Here's how the part is built. I have some questions about the finished solid (model axes, mm). Round coordinates to 2 decimals unless told otherwise and drop trailing zeros. Use one line per item in the form item = value. Start each with the question number.
1. Will these pins go through, and if not, where does the flat tip stop? pin 1 (4 mm diameter, centred on y = 1.5, z = 383, fed in from -X); pin 2 (1.8 mm diameter, centred on x = 2.5, z = 310.5, fed in from +Y); pin 3 (2 mm diameter, centred on x = 4.5, z = 294.5, fed in from -Y).
2. I want a section at A-A, the plane z = 497. State how many separate pieces and enclosed holes the cut face has, plus the area to 3 significant figures.
3. If I drill on line 1 along X through (y, z) = (6.5, 167); line 2 along X through (y, z) = (-1.75, 24.5); line 3 along X through (y, z) = (7.5, 254.5), over which ranges is the centre line in solid material (lowest first)?
```python
from build123d import *

# Parameters (mm, degrees)
EXTRUDE1_DEPTH = 574


with BuildPart() as part:
    # Sketch1 → Extrude1 (new body)
    with BuildSketch(Plane.XY):
        with BuildLine():
            Line((3.232233116, 4.565447254), (0.953589838, 4.565447254))
            ThreePointArc((0.953589838, 4.565447254), (0.901826028, 4.558632419), (0.853589836, 4.538652333))
            Line((0.853589836, 4.538652333), (0.100000003, 4.103567024))
            ThreePointArc((0.100000003, 4.103567024), (0, 4.076772104), (-0.100000003, 4.103567024))
            Line((-0.100000003, 4.103567024), (-0.853589836, 4.538652333))
            ThreePointArc((-0.853589836, 4.538652333), (-0.901826028, 4.558632419), (-0.953589838, 4.565447254))
            Line((-0.953589838, 4.565447254), (-3.232233116, 4.565447254))
            ThreePointArc((-3.232233116, 4.565447254), (-3.417445277, 4.601015929), (-3.576306433, 4.702661433))
            Line((-3.576306433, 4.702661433), (-5.844073317, 6.853456827))
            ThreePointArc((-5.844073317, 6.853456827), (-5.959367314, 7.018804885), (-6, 7.216242649))
            Line((-6, 7.216242649), (-6, 7.948478858))
            ThreePointArc((-6, 7.948478858), (-5.855954134, 8.296236342), (-5.50819665, 8.440282208))
            Line((-5.50819665, 8.440282208), (-3.49180335, 8.440282208))
            ThreePointArc((-3.49180335, 8.440282208), (-3.144045866, 8.584328074), (-3, 8.932085558))
            Line((-3, 8.932085558), (-3, 9.249999634))
            ThreePointArc((-3, 9.249999634), (-3.058578644, 9.39142099), (-3.2, 9.449999634))
            Line((-3.2, 9.449999634), (-3.350000366, 9.449999634))
            ThreePointArc((-3.350000366, 9.449999634), (-3.491421722, 9.508578278), (-3.550000366, 9.649999634))
            Line((-3.550000366, 9.649999634), (-3.550000366, 9.8))
            ThreePointArc((-3.550000366, 9.8), (-3.60857901, 9.941421356), (-3.750000366, 10))
            Line((-3.750000366, 10), (-8.50000115, 10))
            ThreePointArc((-8.50000115, 10), (-9.560660508, 9.560660508), (-10, 8.50000115))
            Line((-10, 8.50000115), (-10, 7))
            ThreePointArc((-10, 7), (-5.02081528, -5.02081528), (7, -10))
            Line((7, -10), (8.50000115, -10))
            ThreePointArc((8.50000115, -10), (9.560660508, -9.560660508), (10, -8.50000115))
            Line((10, -8.50000115), (10, -3.750000366))
            ThreePointArc((10, -3.750000366), (9.941421356, -3.60857901), (9.8, -3.550000366))
            Line((9.8, -3.550000366), (9.649999634, -3.550000366))
            ThreePointArc((9.649999634, -3.550000366), (9.508578278, -3.491421722), (9.449999634, -3.350000366))
            Line((9.449999634, -3.350000366), (9.449999634, -3.2))
            ThreePointArc((9.449999634, -3.2), (9.39142099, -3.058578644), (9.249999634, -3))
            Line((9.249999634, -3), (8.866638303, -3))
            ThreePointArc((8.866638303, -3), (8.518880819, -3.144045866), (8.374834953, -3.49180335))
            Line((8.374834953, -3.49180335), (8.374834953, -5.50819665))
            ThreePointArc((8.374834953, -5.50819665), (8.230789087, -5.855954134), (7.883031603, -6))
            Line((7.883031603, -6), (7.150795394, -6))
            ThreePointArc((7.150795394, -6), (6.95335763, -5.959367314), (6.788009572, -5.844073317))
            Line((6.788009572, -5.844073317), (4.637214178, -3.576306432))
            ThreePointArc((4.637214178, -3.576306432), (4.535568675, -3.417445276), (4.5, -3.232233115))
            Line((4.5, -3.232233115), (4.5, -0.953589838))
            ThreePointArc((4.5, -0.953589838), (4.493185165, -0.901826026), (4.473205078, -0.853589834))
            Line((4.473205078, -0.853589834), (4.038119764, -0.100000004))
            ThreePointArc((4.038119764, -0.100000004), (4.011324842, 0), (4.038119764, 0.100000004))
            Line((4.038119764, 0.100000004), (4.473205078, 0.853589834))
            ThreePointArc((4.473205078, 0.853589834), (4.493185165, 0.901826026), (4.5, 0.953589838))
            Line((4.5, 0.953589838), (4.5, 3.232233115))
            ThreePointArc((4.5, 3.232233115), (4.535568675, 3.417445276), (4.637214178, 3.576306432))
            Line((4.637214178, 3.576306432), (6.788009572, 5.844073317))
            ThreePointArc((6.788009572, 5.844073317), (6.95335763, 5.959367314), (7.150795394, 6))
            Line((7.150795394, 6), (7.883031603, 6))
            ThreePointArc((7.883031603, 6), (8.230789087, 5.855954134), (8.374834953, 5.50819665))
            Line((8.374834953, 5.50819665), (8.374834953, 3.49180335))
            ThreePointArc((8.374834953, 3.49180335), (8.518880819, 3.144045866), (8.866638303, 3))
            Line((8.866638303, 3), (9.249999634, 3))
            ThreePointArc((9.249999634, 3), (9.39142099, 3.058578644), (9.449999634, 3.2))
            Line((9.449999634, 3.2), (9.449999634, 3.350000366))
            ThreePointArc((9.449999634, 3.350000366), (9.508578278, 3.491421722), (9.649999634, 3.550000366))
            Line((9.649999634, 3.550000366), (9.8, 3.550000366))
            ThreePointArc((9.8, 3.550000366), (9.941421356, 3.60857901), (10, 3.750000366))
            Line((10, 3.750000366), (10, 8.50000115))
            ThreePointArc((10, 8.50000115), (9.560660508, 9.560660508), (8.50000115, 10))
            Line((8.50000115, 10), (3.750000366, 10))
            ThreePointArc((3.750000366, 10), (3.60857901, 9.941421356), (3.550000366, 9.8))
            Line((3.550000366, 9.8), (3.550000366, 9.649999634))
            ThreePointArc((3.550000366, 9.649999634), (3.491421722, 9.508578278), (3.350000366, 9.449999634))
            Line((3.350000366, 9.449999634), (3.2, 9.449999634))
            ThreePointArc((3.2, 9.449999634), (3.058578644, 9.39142099), (3, 9.249999634))
            Line((3, 9.249999634), (3, 8.932085558))
            ThreePointArc((3, 8.932085558), (3.144045866, 8.584328074), (3.49180335, 8.440282208))
            Line((3.49180335, 8.440282208), (5.50819665, 8.440282208))
            ThreePointArc((5.50819665, 8.440282208), (5.855954134, 8.296236342), (6, 7.948478858))
            Line((6, 7.948478858), (6, 7.216242649))
            ThreePointArc((6, 7.216242649), (5.959367314, 7.018804885), (5.844073317, 6.853456827))
            Line((5.844073317, 6.853456827), (3.576306433, 4.702661433))
            ThreePointArc((3.576306433, 4.702661433), (3.417445277, 4.601015929), (3.232233116, 4.565447254))
        make_face()
        with BuildLine():
            Line((1.258185436, 2.445295362), (1.887055008, 2.947714945))
            ThreePointArc((1.887055008, 2.947714945), (2.474873794, 2.474873674), (2.947715037, 1.887054865))
            Line((2.947715037, 1.887054865), (2.445295423, 1.258185317))
            ThreePointArc((2.445295423, 1.258185317), (2.75, -6.7e-08), (2.445295362, -1.258185436))
            Line((2.445295362, -1.258185436), (2.947714945, -1.887055008))
            ThreePointArc((2.947714945, -1.887055008), (2.474873674, -2.474873794), (1.887054865, -2.947715037))
            Line((1.887054865, -2.947715037), (1.258185317, -2.445295423))
            ThreePointArc((1.258185317, -2.445295423), (-6.7e-08, -2.75), (-1.258185436, -2.445295362))
            Line((-1.258185436, -2.445295362), (-1.887055008, -2.947714945))
            ThreePointArc((-1.887055008, -2.947714945), (-2.474873794, -2.474873674), (-2.947715037, -1.887054865))
            Line((-2.947715037, -1.887054865), (-2.445295423, -1.258185317))
            ThreePointArc((-2.445295423, -1.258185317), (-2.75, 6.7e-08), (-2.445295362, 1.258185436))
            Line((-2.445295362, 1.258185436), (-2.947714945, 1.887055008))
            ThreePointArc((-2.947714945, 1.887055008), (-2.474873674, 2.474873794), (-1.887054865, 2.947715037))
            Line((-1.887054865, 2.947715037), (-1.258185317, 2.445295423))
            ThreePointArc((-1.258185317, 2.445295423), (6.7e-08, 2.75), (1.258185436, 2.445295362))
        make_face(mode=Mode.SUBTRACT)
        with BuildLine():
            Line((3.232233163, -4.499999714), (-2.000000051, -4.499999587))
            ThreePointArc((-2.000000051, -4.499999587), (-2.474341709, -4.841885693), (-2.300000072, -5.399999581))
            ThreePointArc((-2.300000072, -5.399999581), (1.713541858, -7.57063318), (6.185210557, -8.478569349))
            ThreePointArc((6.185210557, -8.478569349), (6.668243282, -8.182681825), (6.565047479, -7.625707261))
            Line((6.565047479, -7.625707261), (3.585786542, -4.646446324))
            ThreePointArc((3.585786542, -4.646446324), (3.423574873, -4.53805995), (3.232233163, -4.499999714))
        make_face(mode=Mode.SUBTRACT)
        with BuildLine():
            Line((-4.646446492, 3.585787135), (-7.625707283, 6.565048217))
            ThreePointArc((-7.625707283, 6.565048217), (-8.182681843, 6.668244047), (-8.47856939, 6.185211338))
            ThreePointArc((-8.47856939, 6.185211338), (-7.570633447, 1.713542596), (-5.400000054, -2.299999441))
            ThreePointArc((-5.400000054, -2.299999441), (-4.841886176, -2.474341107), (-4.500000045, -1.999999467))
            Line((-4.500000045, -1.999999467), (-4.499999899, 3.232233748))
            ThreePointArc((-4.499999899, 3.232233748), (-4.538060126, 3.42357546), (-4.646446492, 3.585787135))
        make_face(mode=Mode.SUBTRACT)
    extrude(amount=EXTRUDE1_DEPTH)


solid = part.part
```
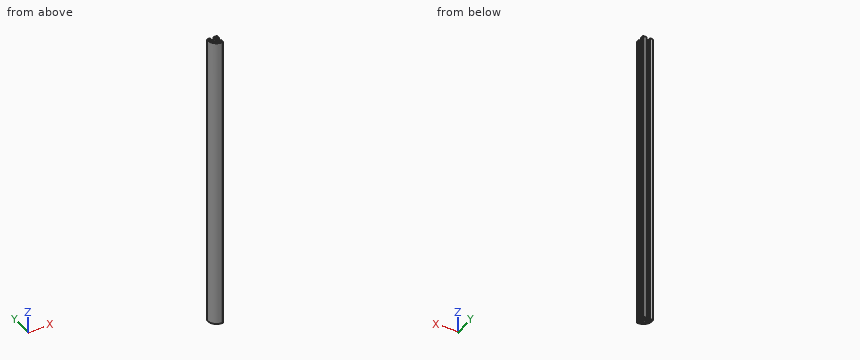
Model answer:
q1.pin_1 = -9.64
q1.pin_2 = 9.46
q1.pin_3 = -9.93
q2.separate_pieces = 1
q2.enclosed_holes = 3
q2.area = 163 mm2
q3.line_1 = -9.99 to -8.39, -7.56 to -5.47, 5.47 to 10
q3.line_2 = -7.58 to -5.79, -4.5 to -2.84, 2.84 to 4.5
q3.line_3 = -10 to -6, 6 to 10
